from build123d import *

# Parameters (mm, degrees)
SKETCH1_W           = 127
SKETCH1_H           = 85
BOSS_EXTRUDE1_DEPTH = 2.5
SKETCH2_W           = 127
SKETCH2_H           = 85
SKETCH2_W_2         = 122
SKETCH2_H_2         = 80
BOSS_EXTRUDE2_DEPTH = 38.5
SKETCH3_W           = 110
SKETCH3_H           = 68.5
CUT_EXTRUDE1_DEPTH  = 2.5
BOSS_EXTRUDE3_DEPTH = 15
SKETCH10_W          = 122
SKETCH10_H          = 2.5
CUT_EXTRUDE2_DEPTH  = 35
SKETCH11_W          = 127
SKETCH11_H          = 41
BOSS_EXTRUDE4_DEPTH = 2.5
CUT_EXTRUDE4_DEPTH  = 2.5
SKETCH14_W          = 15
SKETCH14_H          = 1
CUT_EXTRUDE5_DEPTH  = 1.5
SKETCH13_R          = 1
BOSS_EXTRUDE6_DEPTH = 6
SKETCH17_W          = 12.5
SKETCH17_H          = 8
CUT_EXTRUDE6_DEPTH  = 2.5
SKETCH19_W          = 127
SKETCH19_H          = 102.5
SKETCH19_W_2        = 122
SKETCH19_H_2        = 97.5
BOSS_EXTRUDE7_DEPTH = 4


# Read off the part's stored shape, not the designer's step: #1-64 Machine Threads Stud1
with BuildPart() as part:
    # Sketch1 → Boss-Extrude1 (new body)
    with BuildSketch(Plane(origin=(0, 0, 0), x_dir=(1, 0, 0), z_dir=(0, 1, 0))):
        with Locations((63.5, 42.5)):
            Rectangle(SKETCH1_W, SKETCH1_H)
    extrude(amount=BOSS_EXTRUDE1_DEPTH)

    # Sketch2 → Boss-Extrude2 (add)
    with BuildSketch(Plane(origin=(0, 2.5, 0), x_dir=(1, 0, 0), z_dir=(0, 1, 0))):
        with Locations((63.5, 42.5)):
            Rectangle(SKETCH2_W, SKETCH2_H)
        with Locations((63.5, 42.5)):
            Rectangle(SKETCH2_W_2, SKETCH2_H_2, mode=Mode.SUBTRACT)
    extrude(amount=BOSS_EXTRUDE2_DEPTH)

    # Sketch3 → Cut-Extrude1 (cut)
    with BuildSketch(Plane(origin=(0, 0, 0), x_dir=(-1, 0, 0), z_dir=(0, -1, 0))):
        with Locations((-63.5, 39.75)):
            Rectangle(SKETCH3_W, SKETCH3_H)
    extrude(amount=-CUT_EXTRUDE1_DEPTH, mode=Mode.SUBTRACT)

    # Sketch9 → Boss-Extrude3 (add)
    with BuildSketch(Plane(origin=(0, 0, -85), x_dir=(-1, 0, 0), z_dir=(0, 0, -1))):
        Polygon((-127, 0), (0, 0), (0, 2.5), (0, 41), (-2.5, 41), (-2.5, 2.5), (-124.5, 2.5), (-124.5, 41), (-127, 41), (-127, 2.5), align=None)
    extrude(amount=BOSS_EXTRUDE3_DEPTH)

    # Sketch10 → Cut-Extrude2 (cut)
    with BuildSketch(Plane(origin=(0, 41, 0), x_dir=(1, 0, 0), z_dir=(0, 1, 0))):
        with Locations((63.5, 83.75)):
            Rectangle(SKETCH10_W, SKETCH10_H)
    extrude(amount=-CUT_EXTRUDE2_DEPTH, mode=Mode.SUBTRACT)

    # Sketch11 → Boss-Extrude4 (add)
    with BuildSketch(Plane(origin=(0, 0, -100), x_dir=(-1, 0, 0), z_dir=(0, 0, -1))):
        with Locations((-63.5, 20.5)):
            Rectangle(SKETCH11_W, SKETCH11_H)
    extrude(amount=BOSS_EXTRUDE4_DEPTH)

    # Sketch6 → Cut-Extrude4 (cut)
    with BuildSketch(Plane(origin=(0, 0, 0), x_dir=(-1, 0, 0), z_dir=(0, -1, 0))):
        with BuildLine():
            Line((-61.1, 90.153713072), (-65.9, 90.153713072))
            ThreePointArc((-65.9, 90.153713072), (-68.4, 92.653713072), (-65.9, 95.153713072))
            Line((-65.9, 95.153713072), (-61.1, 95.153713072))
            ThreePointArc((-61.1, 95.153713072), (-58.6, 92.653713072), (-61.1, 90.153713072))
        make_face()
    extrude(amount=-CUT_EXTRUDE4_DEPTH, mode=Mode.SUBTRACT)

    # Sketch14 → Cut-Extrude5 (cut)
    with BuildSketch(Plane(origin=(0, 2.5, 0), x_dir=(1, 0, 0), z_dir=(0, 1, 0))):
        with Locations((63.5, 86.653713072)):
            Rectangle(SKETCH14_W, SKETCH14_H)
    extrude(amount=-CUT_EXTRUDE5_DEPTH, mode=Mode.SUBTRACT)

    # Sketch13 → Boss-Extrude6 (add)
    with BuildSketch(Plane(origin=(0, 2.5, 0), x_dir=(1, 0, 0), z_dir=(0, 1, 0))):
        with Locations((56.3, 92.653713072)):
            Circle(SKETCH13_R)
        with Locations((70.7, 92.653713072)):
            Circle(SKETCH13_R)
    extrude(amount=BOSS_EXTRUDE6_DEPTH)

    # Sketch17 → Cut-Extrude6 (cut)
    with BuildSketch(Plane.XY):
        with Locations((45.75, 22.5)):
            Rectangle(SKETCH17_W, SKETCH17_H)
    extrude(amount=-CUT_EXTRUDE6_DEPTH, mode=Mode.SUBTRACT)

    # Sketch19 → Boss-Extrude7 (add)
    with BuildSketch(Plane(origin=(0, 41, 0), x_dir=(1, 0, 0), z_dir=(0, 1, 0))):
        with Locations((63.5, 51.25)):
            Rectangle(SKETCH19_W, SKETCH19_H)
        with Locations((63.5, 51.25)):
            Rectangle(SKETCH19_W_2, SKETCH19_H_2, mode=Mode.SUBTRACT)
    extrude(amount=BOSS_EXTRUDE7_DEPTH)

    # #1-64 Machine Threads Stud1 outline → #1-64 Machine Threads Stud1 (revolve, cut)
    with BuildSketch(Plane(origin=(70.7, 0, -92.653713072), x_dir=(1, 0, 0), z_dir=(0, 0, 1))):
        Polygon((1, 8.5), (0.69088, 8.5), (0.9271, 8.26378), (0.9271, 2.5), (1, 2.5), align=None)
    revolve(axis=Axis((70.7, 0, -92.653713072), (0, 1, 0)), mode=Mode.SUBTRACT)


solid = part.part
Can you work these out from the model? Positions are in its coordinate system, mm. A direction names the side the tool comes from. Give positions to 0.01 mm unless a question says otherwise; leave off trailing zeros. Order: outer loops, then holes, each group sorted by start corner. A loop starts at its lowest first (then second) coordinate and runs counter-clockwise, first axis right, second up. Notation, with made-up numbers: M -18.75,28 L 38.25,28 A25 ccw 38.25,54 Z; hole C 49.5,56.25 d7. An arc over 180 degrees is marked long. Use one line per item in the form item = value. Start each with the question number.
Item 1: If we section it at D-D (z = -11): Write out the boundary of the cut face in (x, y), then the cut area to 3 significant figures.
Item 2: For faces 4 (the flat face through (63, 2.5, -96)), 5 (the flat face through (0, 22, -51)), which set-ups out of +Z, -Z, +X, -X, +Y, -Y let a thin tool reach every point of the face, with its end or its side?
Item 3: If I drill on line 1 along X through (y, z) = (17, -70); line 2 along Z through (x, y) = (117, 39); line 3 along Z through (x, y) = (41, 26), over which ranges is the centre line in solid material (lowest first)?
Item 4: If we section it at C-C (y = 35): Write out the boundary of the cut face in (x, z).
Item 5: Will these pins go through, and if not, where does the flat tip stop? pin 1 Ø5 at (y, z) = (40, -56.5) entering from -X; pin 2 Ø4.5 at (x, z) = (86.5, -89.5) entering from +Y; pin 3 Ø0.8 at (x, z) = (81.5, -83.5) entering from +Y; pin 4 Ø0.6 at (x, z) = (56, -93) entering from +Y.
Item 6: If we section it at B-B (z = -78): Write out the boundary of the cut face in (x, y).
Item 7: We'd pull the mould along Z, two halves only. Please class faces 1 (the flat face through (64, 0, -85)), 2 (the flat face through (63, 23, -100)), 3 (the flat face through (63, 22, -102.5)): +Z half, -Z half, draft (parallel to the pull), parting line (faces both ways), or undercut.
Item 8: If we section it at A-A (x = 73): Write out the boundary of the cut face in (y, z).
Outcome:
q1.outline = M 0,0 L 8.5,0 L 8.5,2.5 L 2.5,2.5 L 2.5,45 L 0,45 Z; M 118.5,0 L 127,0 L 127,45 L 124.5,45 L 124.5,2.5 L 118.5,2.5 Z
q1.area = 255 mm2
q2.face_4 = +Y
q2.face_5 = +Z, -Z, -X, +Y, -Y
q3.line_1 = 0 to 2.5, 124.5 to 127
q3.line_2 = -102.5 to -100, -2.5 to 0
q3.line_3 = -102.5 to -100
q4.outline = M 0,-102.5 L 127,-102.5 L 127,0 L 0,0 Z; hole M 2.5,-100 L 124.5,-100 L 124.5,-2.5 L 2.5,-2.5 Z
q5.pin_1 = 0
q5.pin_2 = 2.5
q5.pin_3 = 6
q5.pin_4 = 8.5
q6.outline = M 0,0 L 127,0 L 127,45 L 124.5,45 L 124.5,2.5 L 2.5,2.5 L 2.5,45 L 0,45 Z
q7.face_1 = draft
q7.face_2 = undercut
q7.face_3 = -Z half
q8.outline = M 0,-102.5 L 45,-102.5 L 45,-100 L 2.5,-100 L 2.5,-85 L 6,-85 L 6,-82.5 L 2.5,-82.5 L 2.5,-74 L 0,-74 Z; M 0,-5.5 L 2.5,-5.5 L 2.5,-2.5 L 45,-2.5 L 45,0 L 0,0 Z
